Autodesk Inventor part; units mm, degrees
ref_plane "YZ Plane" through (0, 0, 0) normal (1, 0, 0) x (0, 1, 0)
ref_plane "XZ Plane" through (0, 0, 0) normal (0, 1, 0) x (-1, 0, 0)
ref_plane "XY Plane" through (0, 0, 0) normal (0, 0, 1) x (1, 0, 0)
sketch "草图1" plane through (0, 0, 0) normal (0, 0, 1) x (1, 0, 0)
  circle A0 centre (37.7249, -83) radius 3.6
  line L0 (65, -83) -> (65, -51)
  line L1 (65, -51) -> (47, -51)
  line L2 (47, -51) -> (47, -83)
  line L3 (47, -83) -> (65, -83)
  line L4 (89.2, -11.5) -> (96, -11.5)
  line L5 (96, -25) -> (96, -11.5)
  line L6 (96, -25) -> (101, -25)
  line L7 (101, -25) -> (101, -45)
  line L8 (96, -45) -> (101, -45)
  line L9 (96, -58.5) -> (96, -45)
  line L10 (96, -58.5) -> (89.2, -58.5)
  line L11 (89.2, -58.5) -> (89.2, -56.75)
  line L12 (89.2, -56.75) -> (86.8, -56.75)
  line L13 (86.8, -56.75) -> (86.8, -58.5)
  line L14 (86.8, -58.5) -> (84, -58.5)
  line L15 (84, -58.5) -> (84, -61.5)
  line L16 (84, -61.5) -> (86.8, -61.5)
  line L17 (86.8, -61.5) -> (86.8, -63.25)
  line L18 (86.8, -63.25) -> (89.2, -63.25)
  line L19 (89.2, -63.25) -> (89.2, -61.5)
  line L20 (89.2, -61.5) -> (96, -61.5)
  line L21 (96, -75) -> (96, -61.5)
  line L22 (96, -75) -> (101, -75)
  line L23 (101, -75) -> (101, -100)
  line L24 (101, -100) -> (63, -100)
  line L25 (63, -95) -> (63, -100)
  line L26 (33, -95) -> (63, -95)
  line L27 (33, -95) -> (33, -100)
  line L28 (33, -100) -> (-5, -100)
  line L29 (-5, -75) -> (-5, -100)
  line L30 (0, -75) -> (-5, -75)
  line L31 (0, -75) -> (0, -61.5)
  line L32 (0, -61.5) -> (6.8, -61.5)
  line L33 (6.8, -61.5) -> (6.8, -63.25)
  line L34 (6.8, -63.25) -> (9.2, -63.25)
  line L35 (9.2, -63.25) -> (9.2, -61.5)
  line L36 (9.2, -61.5) -> (12, -61.5)
  line L37 (12, -61.5) -> (12, -58.5)
  line L38 (12, -58.5) -> (9.2, -58.5)
  line L39 (9.2, -58.5) -> (9.2, -56.75)
  line L40 (9.2, -56.75) -> (6.8, -56.75)
  line L41 (6.8, -56.75) -> (6.8, -58.5)
  line L42 (6.8, -58.5) -> (0, -58.5)
  line L43 (0, -58.5) -> (0, -45)
  line L44 (0, -45) -> (-5, -45)
  line L45 (-5, -45) -> (-5, -25)
  line L46 (0, -25) -> (-5, -25)
  line L47 (0, -25) -> (0, -11.5)
  line L48 (0, -11.5) -> (6.8, -11.5)
  line L49 (6.8, -11.5) -> (6.8, -13.25)
  line L50 (6.8, -13.25) -> (9.2, -13.25)
  line L51 (9.2, -13.25) -> (9.2, -11.5)
  line L52 (9.2, -11.5) -> (12, -11.5)
  line L53 (12, -11.5) -> (12, -8.5)
  line L54 (12, -8.5) -> (9.2, -8.5)
  line L55 (9.2, -8.5) -> (9.2, -6.75)
  line L56 (9.2, -6.75) -> (6.8, -6.75)
  line L57 (6.8, -6.75) -> (6.8, -8.5)
  line L58 (6.8, -8.5) -> (0, -8.5)
  line L59 (0, -8.5) -> (0, 5)
  line L60 (0, 5) -> (-5, 5)
  line L61 (-5, 5) -> (-5, 26)
  line L62 (33, 26) -> (-5, 26)
  line L63 (33, 21) -> (33, 26)
  line L64 (33, 21) -> (46.5, 21)
  line L65 (46.5, 21) -> (46.5, 14.2)
  line L66 (46.5, 14.2) -> (44.75, 14.2)
  line L67 (44.75, 14.2) -> (44.75, 11.8)
  line L68 (44.75, 11.8) -> (46.5, 11.8)
  line L69 (46.5, 11.8) -> (46.5, 9)
  line L70 (46.5, 9) -> (49.5, 9)
  line L71 (49.5, 9) -> (49.5, 11.8)
  line L72 (49.5, 11.8) -> (51.25, 11.8)
  line L73 (51.25, 11.8) -> (51.25, 14.2)
  line L74 (51.25, 14.2) -> (49.5, 14.2)
  line L75 (49.5, 14.2) -> (49.5, 21)
  line L76 (49.5, 21) -> (63, 21)
  line L77 (63, 21) -> (63, 26)
  line L78 (63, 26) -> (101, 26)
  line L79 (101, 26) -> (101, 5)
  line L80 (96, 5) -> (101, 5)
  line L81 (96, -8.5) -> (96, 5)
  line L82 (96, -8.5) -> (89.2, -8.5)
  line L83 (89.2, -8.5) -> (89.2, -6.75)
  line L84 (89.2, -6.75) -> (86.8, -6.75)
  line L85 (86.8, -6.75) -> (86.8, -8.5)
  line L86 (86.8, -8.5) -> (84, -8.5)
  line L87 (84, -8.5) -> (84, -11.5)
  line L88 (84, -11.5) -> (86.8, -11.5)
  line L89 (86.8, -11.5) -> (86.8, -13.25)
  line L90 (86.8, -13.25) -> (89.2, -13.25)
  line L91 (89.2, -13.25) -> (89.2, -11.5)
  line L92 (25, 0) -> (25, 5)
  line L93 (25, 5) -> (5, 5)
  line L94 (5, 5) -> (5, 0)
  line L95 (5, 0) -> (25, 0)
  line L96 (28, -35) -> (28, -50)
  line L97 (28, -50) -> (33, -50)
  line L98 (33, -50) -> (33, -35)
  line L99 (33, -35) -> (28, -35)
  line L100 (28, -5) -> (28, -20)
  line L101 (28, -20) -> (33, -20)
  line L102 (33, -20) -> (33, -5)
  line L103 (33, -5) -> (28, -5)
  line L104 (46, -42) -> (46, -47)
  line L105 (46, -47) -> (61, -47)
  line L106 (61, -47) -> (61, -42)
  line L107 (61, -42) -> (46, -42)
  line L108 (76, -42) -> (76, -47)
  line L109 (76, -47) -> (91, -47)
  line L110 (91, -47) -> (91, -42)
  line L111 (91, -42) -> (76, -42)
  circle A1 centre (66, -9) radius 3
  point P0 (0, 0)
extrude "拉伸1" add sketch "草图1" along normal blind 5 contours A0 | L3 L2 L1 L0 | L4 L5 L6 L7 L8 L9 L10 L11 L12 L13 L14 L15 L16 L17 L18 L19 L20 L21 L22 L23 L24 L25 L26 L27 L28 L29 L30 L31 L32 L33 L34 L35 L36 L37 L38 L39 L40 L41 L42 L43 L44 L45 L46 L47 L48 L49 L50 L51 L52 L53 L54 L55 L56 L57 L58 L59 L60 L61 L62 L63 L64 L65 L66 L67 L68 L69 L70 L71 L72 L73 L74 L75 L76 L77 L78 L79 L80 L81 L82 L83 L84 L85 L86 L87 L88 L89 L90 L91
sketch "草图2" plane through (0, 0, 5) normal (0, 0, 1) x (1, 0, 0)
  circle A0 centre (66, -9) radius 3
  line L0 (96, -25) -> (96, -11.5)
  circle A1 centre (55.0452, -9) radius 6
  line L1 (60.2413, -12) -> (66, -12)
  line L2 (60.2413, -6) -> (66, -6)
  point P0 (0, 0)
  dimension "d2" = 12
extrude "拉伸2" cut sketch "草图2" against normal through all contours A0 L1 A1 L2 | A1
properties part number "left"
Here's how the part is built. I have some questions about the finished solid (model axes, mm). A direction names the side the tool comes from. Give positions to 0.01 mm unless a question says otherwise; leave off trailing zeros. Write each loop counter-clockwise with the first axis right and the second up, starting at its lowest first coordinate (ties: lowest second). Pieces come first, ordered by that corner, then holes. Notation, with made-up numbers: M 54,5 L 72,5 A23 ccw 72,14 Z; hole C 71.5,-2.5 d10. An arc over 180 degrees is marked long. Put each result on its own line as item: value. Start each with the question number.
Item 1: If we section it at A-A, the plane y = 16: Write out the boundary of the cut face in (x, z), then the cut area to 3 significant figures.
Item 2: If we section it at C-C, the plane y = -65: Write out the boundary of the cut face in (x, z).
Item 3: Thinking about a two-plate mould opening in Y: for faces 1 (the flat face through (98, -75, 2)), 2 (the flat face through (46.5, 10, 2)), 3 (the flat face through (48, -95, 2)), which applies, +Y half, -Y half, draft (parallel to the pull), parting line (faces both ways), or undercut?
Item 4: I need wall thicknesses on L1, parallel to X at y = -9, z = 3.35; L2, parallel to X at y = 10, z = 1.5; L3, parallel to Y at x = 8, z = 3.4. Which ranges of each line are inside material? Lowest first, please. Write a range as from..to.
Item 5: If we section it at B-B, the plane x = 80.5: Write out the boundary of the cut face in (y, z).
Item 6: On a 3-axis mill with a long thin cutter (end or side, diameter ignored), from which of +Z, -Z, +X, -X, +Y, -Y can I reach the whole of each face in a straight line? I mean faces 4 (the flat face through (47, -36, 0)), 5 (the flat face through (0, -52, 2)), 6 (the flat face through (56, 21, 2)), 7 (the flat face through (91, -45, 2)), 8 (the flat face through (85, -58.5, 2)). Say none if no direction works.
Item 7: If we section it at D-D, the plane z = 1.7: Count the separate pieces of the cut face and the enclosed holes in it, then the cut area to 3 significant figures.
Item 8: Will these pins go through, and if not, where does the flat tip stop? pin 1 (1 mm diameter, centred on y = -56, z = 3, fed in from +X); pin 2 (12 mm diameter, centred on x = 30, y = -13.5, fed in from -Z); pin 3 (0.9 mm diameter, centred on x = 47.5, z = 3.5, fed in from +Y); pin 4 (2.5 mm diameter, centred on x = 42.5, z = 3.5, fed in from +Y).
Values:
1. outline: M -5,0 L 46.5,0 L 46.5,5 L -5,5 Z; M 49.5,0 L 101,0 L 101,5 L 49.5,5 Z
1. area: 515 mm²
2. outline: M 0,0 L 96,0 L 96,5 L 0,5 Z
3. face 1: undercut
3. face 2: draft
3. face 3: -Y half
4. L1: 12..28, 33..49.05, 69..84
4. L2: -5..46.5, 49.5..101
4. L3: -100..-63.25, -56.75..-13.25, -6.75..0, 5..26
5. outline: M -100,0 L -47,0 L -47,5 L -100,5 Z; M -42,0 L 26,0 L 26,5 L -42,5 Z
6. face 4: -Z, +X, -X, +Y, -Y
6. face 5: +Z, -Z, -X
6. face 6: +Z, -Z, +Y
6. face 7: +Z, -Z
6. face 8: +Z, -Z, +X
7. separate pieces: 1
7. enclosed holes: 6
7. area: 11,700 mm²
8. pin 1: x = 96
8. pin 2: z = 0
8. pin 3: y = 9
8. pin 4: y = 21
